Can you work these out from the drawing? Everything is in mm from the part's minimum corner. Round coordinates to 2 decimals unless told otherwise and drop trailing zeros. Order: outer loops, then holes, each group sorted by start corner. A loop starts at its lowest first (then second) coordinate and runs counter-clockwise, first axis right, second up. Notation, with made-up numbers: M 70,87 L 95,87 A16 cw 95,105 Z; hole C 42.25,37.25 d10. An arc over 180 degrees is marked long. Write item = value, one per line. Start each with the question number.
Item 1: I'm going to push flat-ended pins straight in: P1, Ø1.5, axis at x = 2, z = 12, coming from the +Y side; P2, Ø1, axis at x = 3.5, z = 5.5, coming from the -Y side. Where does each tip first touch, or does it pass through?
Item 2: I want a section at D-D, the plane z = 9.5. List the corners of the cut face in (x, y) for me, plus the area to 3 significant figures.
Item 3: I want a section at A-A, the plane z = 7.5. List the corners of the cut face in (x, y) for me.
Item 4: Please list where these lines run through material, in increasing order: L1, parallel to Y at x = 1.85, z = 8.25 (1 decimal); L2, parallel to Y at x = 0.7, z = 9 (1 decimal); L3, parallel to Z at x = 3.4, y = 18.75.
Item 5: I want a section at C-C, the plane x = 1.5. List the corners of the cut face in (y, z) for me (1 decimal).
Item 6: I want a section at B-B, the plane y = 19. List the corners of the cut face in (x, z) for me.
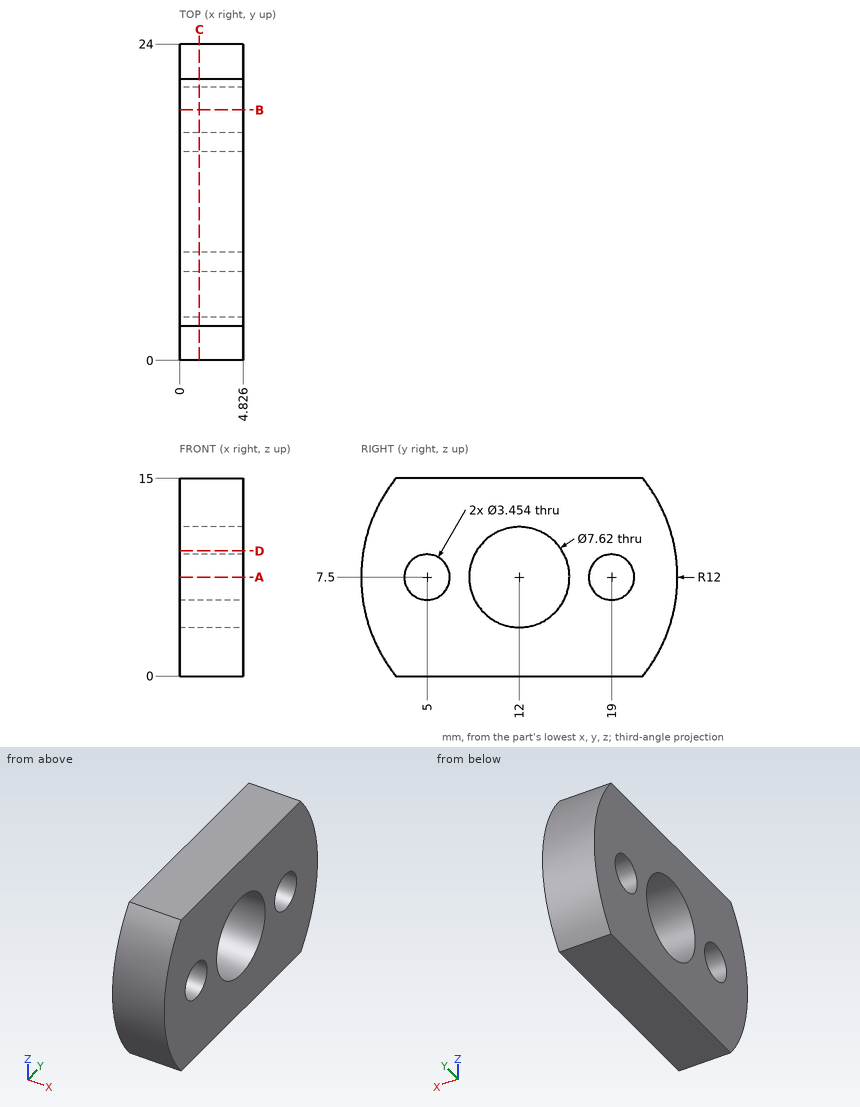
Filled in:
q1.P1 = 23.4
q1.P2 = 0.09
q2.outline = M 0,0.17 L 4.83,0.17 L 4.83,8.76 L 0,8.76 Z; M 0,15.24 L 4.83,15.24 L 4.83,23.83 L 0,23.83 Z
q2.area = 82.9 mm^2
q3.outline = M 0,0 L 4.83,0 L 4.83,3.27 L 0,3.27 Z; M 0,6.73 L 4.83,6.73 L 4.83,8.19 L 0,8.19 Z; M 0,15.81 L 4.83,15.81 L 4.83,17.27 L 0,17.27 Z; M 0,20.73 L 4.83,20.73 L 4.83,24 L 0,24 Z
q4.L1 = 0 to 3.4, 6.6 to 8.3, 15.7 to 17.4, 20.6 to 24
q4.L2 = 0.1 to 4.1, 5.9 to 8.5, 15.5 to 18.1, 19.9 to 23.9
q4.L3 = 0 to 5.79, 9.21 to 15
q5.outline = M 2.6,0 L 21.4,0 A12 ccw 21.4,15 L 2.6,15 A12 ccw Z; hole C 5,7.5 d3.5; hole C 12,7.5 d7.6; hole C 19,7.5 d3.5
q6.outline = M 0,0 L 4.83,0 L 4.83,5.77 L 0,5.77 Z; M 0,9.23 L 4.83,9.23 L 4.83,15 L 0,15 Z
